Source: CAD feature listing. Evaluate the final solid. Frame: model axes, mm. Face numbers are marked on the shaded views. A direction names the side the tool comes from. Round coordinates to 2 decimals unless told otherwise and drop trailing zeros. Write each loop counter-clockwise with the first axis right and the second up, starting at its lowest first coordinate (ties: lowest second). Pieces come first, ordered by that corner, then holes.
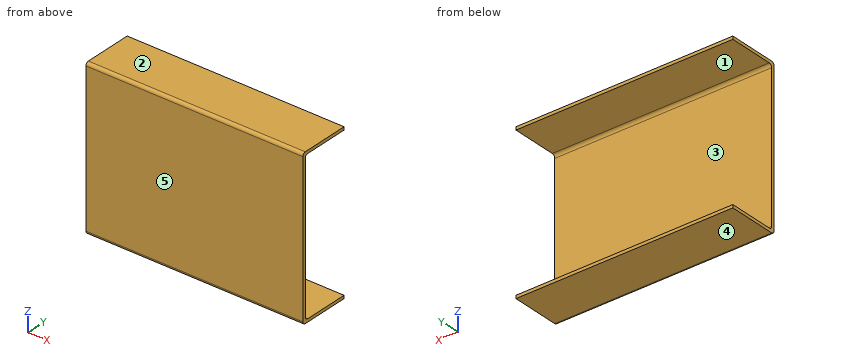
Autodesk Inventor part; units mm, degrees
ref_plane "YZ Plane" through (0, 0, 0) normal (1, 0, 0) x (0, 1, 0)
ref_plane "XZ Plane" through (0, 0, 0) normal (0, 1, 0) x (-1, 0, 0)
ref_plane "XY Plane" through (0, 0, 0) normal (0, 0, 1) x (1, 0, 0)
sketch "Sketch1" plane through (0, 0, 0) normal (1, 0, 0) x (0, 1, 0)
  line L0 (0, 0) -> (-50.8, 0)
  line L1 (-53.975, -3.175) -> (-53.975, -161.925)
  line L2 (-50.8, -165.1) -> (0, -165.1)
  line L3 (0, -161.925) -> (-47.625, -161.925)
  line L4 (-50.8, -158.75) -> (-50.8, -6.35)
  line L5 (-47.625, -3.175) -> (0, -3.175)
  line L6 (0, 0) -> (0, -3.175)
  line L7 (0, -161.925) -> (0, -165.1)
  arc A0 (-50.8, 0) -> (-53.975, -3.175) centre (-50.8, -3.175) ccw
  arc A1 (-53.975, -161.925) -> (-50.8, -165.1) centre (-50.8, -161.925) ccw
  arc A2 (-47.625, -3.175) -> (-50.8, -6.35) centre (-47.625, -6.35) ccw
  arc A3 (-50.8, -158.75) -> (-47.625, -161.925) centre (-47.625, -158.75) ccw
  point P0 (-50.8, -161.925)
  point P1 (-50.8, -3.175)
  dimension "d3" = 3.175
  dimension "d4" = 50.8
  dimension "d5" = 158.75
  dimension "d6" = 3.175
extrude "Extrusion1" add sketch "Sketch1" along normal blind 228.6
properties part number "improved lift c chanel"
1) Pull-direction query (Z, two-part tool) for the marked faces 3, 4 and 5; classes: released by +Z, released by -Z, zero draft, split by the parting line, or undercut.
Taken from the geometry:
face 3: undercut
face 4: released by -Z
face 5: zero draft
2) Reachability of the marked faces 1 and 2 from +Z, -Z, +X, -X, +Y, -Y: full face, straight path, thin tool, end or side. Return the list, or none.
Taken from the geometry:
face 1: +X, -X, +Y
face 2: +Z, +X, -X, +Y, -Y
3) Section query A-A on y = -29.5. Return the cut outline in (x, z) (3 decimals).
Taken from the geometry:
outline: (0, -165.1) - (228.6, -165.1) - (228.6, -161.925) - (0, -161.925) - close; (0, -3.175) - (228.6, -3.175) - (228.6, 0) - (0, 0) - close
4) Contact query for a flat-ended pin moving along its axis: P1, Ø10, axis at x = 116, z = -96.5, coming from the +Y side. Output: stop coordinate, or through.
Taken from the geometry:
P1: stops at y = -50.8
5) Material intervals for line 1 (Z direction, x = 201.5, y = -33) (3 decimals); line 2 (Y direction, x = 108, z = -41) (3 decimals); line 3 (Z direction, x = 101, y = -51), sorted ascending.
Taken from the geometry:
line 1: z = -165.1 to -161.925, -3.175 to 0
line 2: y = -53.975 to -50.8
line 3: z = -165.09 to -0.01
6) Section query B-B on x = 211.5. Return the cut outline in (y, z) (3 decimals).
Taken from the geometry:
outline: (-53.975, -161.925) arc R3.175 ccw to (-50.8, -165.1) - (0, -165.1) - (0, -161.925) - (-47.625, -161.925) arc R3.175 cw to (-50.8, -158.75) - (-50.8, -6.35) arc R3.175 cw to (-47.625, -3.175) - (0, -3.175) - (0, 0) - (-50.8, 0) arc R3.175 ccw to (-53.975, -3.175) - close
7) Section query C-C on z = -30. Return the cut outline in (x, y) (3 decimals), then the cut area to 3 significant figures.
Taken from the geometry:
outline: (0, -53.975) - (228.6, -53.975) - (228.6, -50.8) - (0, -50.8) - close
area: 726 mm2
